Read the model definition and answer for the solid it produces. Units are mm, in the model's axes. Face numbers are marked on the shaded views. A direction names the side the tool comes from. Round coordinates to 2 decimals unless told otherwise and drop trailing zeros. Order: outer loops, then holes, each group sorted by start corner. A loop starts at its lowest first (then second) coordinate and runs counter-clockwise, first axis right, second up. Notation, with made-up numbers: (15, 59) - (47, 59) arc R20 ccw to (47, 68) - close; hole circle Ø8 at (6.25, -23.75). An arc over 180 degrees is marked (long way). Put each result on its own line as item: value. Start each with the question number.
Q1. Which of the six approach directions +Z, -Z, +X, -X, +Y, -Y give full straight-line access (tool end or side, diameter ignored) to the marked faces 5 and 6?
Q2. Find the intervals of material crossed by line 1 along Y through (x, z) = (-19, 70); line 2 along X through (y, z) = (41.5, 50); line 3 along Z through (x, y) = (95, -32), in increasing order. Write a range as from..to.
Q3. Each of these flat-tipped pins is pushed along its axis until it touches: pin 1 Ø2 at (x, z) = (14, 73.5) entering from -Y; pin 2 Ø12 at (x, y) = (8.5, -19) entering from +Z; pin 3 Ø2 at (y, z) = (37.5, 74.5) entering from +X. Where does it stop, or does it pass through?
Q4. For a pull along X with two mould halves and no side action, classify the marked faces 1, 2, 3 and 4 as pulls with the +X half, pulls with the -X half, needs draft (parallel to the pull), parting line crosses it, or undercut.
Q5. Section B-B on z = 27.5 is taken. Give the vertices of the cut face in (x, y), then the cut area to 3 significant figures.
Q6. Section A-A on x = 114.5 is taken. Give the vertices of the cut face in (y, z), then the cut area to 3 significant figures.
Q7. Section C-C on y = -28 is taken. Give the vertices of the cut face in (x, z).
from build123d import *

# Parameters (mm, degrees)
F0_W     = 155.229896307
F0_H     = 82.4026092887
F1_DEPTH = 75.438
F2_DEPTH = 77.216
F3_DEPTH = 96.012
F4_R     = 5.08
F5_T     = -2.54
F6_R     = 16.8009840587
F7_DEPTH = 2.54


# Not quite as in the source:
# - a shell that OpenCascade refuses in one call is made with other operations: the cavity is built on its own and cut out


with BuildPart() as f1:
    # F0 (on Top) → F1 (new body)
    with BuildSketch(Plane.XY):
        with Locations((77.6149481535, 41.2013046443)):
            Rectangle(F0_W, F0_H)
    extrude(amount=F1_DEPTH)

    # F2 (add): a face of the model
    f2_faces = [f1.faces().sort_by_distance(p)[0] for p in [
        (77.6149481535, 0, 37.719),
    ]]
    extrude(f2_faces, amount=F2_DEPTH)

    # F3 (add): a face of the model
    f3_faces = [f1.faces().sort_by_distance(p)[0] for p in [
        (0, 2.5933046443, 37.719),
    ]]
    extrude(f3_faces, amount=F3_DEPTH)

    # F4
    f4_edges = [f1.edges().sort_by_distance(p)[0] for p in [
        (-96.012, 2.593305, 75.438),
        (29.608948, -77.216, 75.438),
        (29.608948, -77.216, 0),
        (-96.012, -77.216, 37.719),
        (-96.012, 2.593305, 0),
        (29.608948, 82.402609, 75.438),
        (155.229896, 2.593305, 75.438),
        (155.229896, -77.216, 37.719),
        (-96.012, 82.402609, 37.719),
        (29.608948, 82.402609, 0),
        (155.229896, 82.402609, 37.719),
        (155.229896, 2.593305, 0),
    ]]
    fillet(f4_edges, radius=F4_R)

    # F5: a shell. OpenCascade refuses it in one call, so the cavity is built on its own and cut out:
    # the body offset inwards by the wall thickness, plus a prism from it out through each open face.
    f5_core = offset(f1.part, amount=F5_T, mode=Mode.PRIVATE)
    f5_exits = [f5_core.faces().sort_by_distance(p)[0] for p in [
        (29.608948, 2.593305, 72.898),
    ]]
    add(f5_core, mode=Mode.SUBTRACT)
    extrude(f5_exits, amount=-F5_T, mode=Mode.SUBTRACT)

    # F6 (on face) → F7 (join, through all)
    with BuildSketch(Plane.YZ.offset(155.229896307)):
        with Locations((0, 37.719)):
            Circle(F6_R)
    extrude(amount=-F7_DEPTH)


solid = f1.part
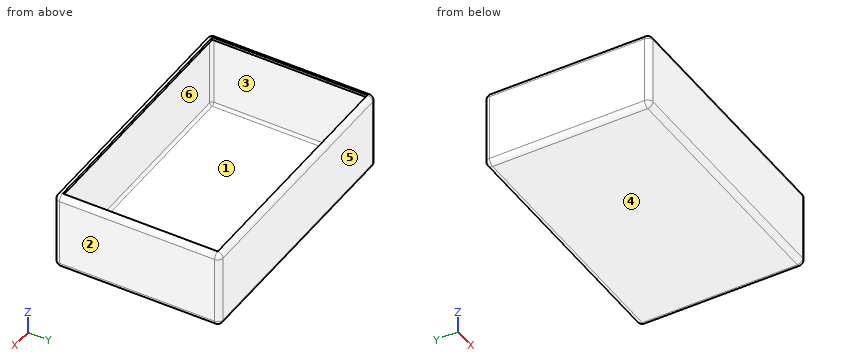
Findings:
1. face 5: +Z, -Z, +X, -X, +Y
1. face 6: none
2. line 1: -77.22..-74.68, 79.86..82.4
2. line 2: -96.01..-93.47, 152.69..155.23
2. line 3: 0..2.54
3. pin 1: y = -76.74
3. pin 2: z = 2.54
3. pin 3: x = 154.14
4. face 1: undercut
4. face 2: pulls with the +X half
4. face 3: undercut
4. face 4: needs draft
5. outline: (-96.01, -72.14) arc R5.08 ccw to (-90.93, -77.22) - (150.15, -77.22) arc R5.08 ccw to (155.23, -72.14) - (155.23, 77.32) arc R5.08 ccw to (150.15, 82.4) - (-90.93, 82.4) arc R5.08 ccw to (-96.01, 77.32) - close; hole (-93.47, -72.14) arc R2.54 ccw to (-90.93, -74.68) - (150.15, -74.68) arc R2.54 ccw to (152.69, -72.14) - (152.69, 77.32) arc R2.54 ccw to (150.15, 79.86) - (-90.93, 79.86) arc R2.54 ccw to (-93.47, 77.32) - close
5. area: 2,040 mm2
6. outline: (-77.22, 5.08) arc R5.08 ccw to (-72.14, 0) - (77.32, 0) arc R5.08 ccw to (82.4, 5.08) - (82.4, 70.36) arc R5.08 ccw to (77.32, 75.44) - (77.32, 72.9) arc R2.54 cw to (79.86, 70.36) - (79.86, 5.08) arc R2.54 cw to (77.32, 2.54) - (-72.14, 2.54) arc R2.54 cw to (-74.68, 5.08) - (-74.68, 70.36) arc R2.54 cw to (-72.14, 72.9) - (-72.14, 75.44) arc R5.08 ccw to (-77.22, 70.36) - close
6. area: 772 mm2
7. outline: (-96.01, 5.08) arc R5.08 ccw to (-90.93, 0) - (150.15, 0) arc R5.08 ccw to (155.23, 5.08) - (155.23, 70.36) arc R5.08 ccw to (150.15, 75.44) - (150.15, 72.9) arc R2.54 cw to (152.69, 70.36) - (152.69, 5.08) arc R2.54 cw to (150.15, 2.54) - (-90.93, 2.54) arc R2.54 cw to (-93.47, 5.08) - (-93.47, 70.36) arc R2.54 cw to (-90.93, 72.9) - (-90.93, 75.44) arc R5.08 ccw to (-96.01, 70.36) - close
